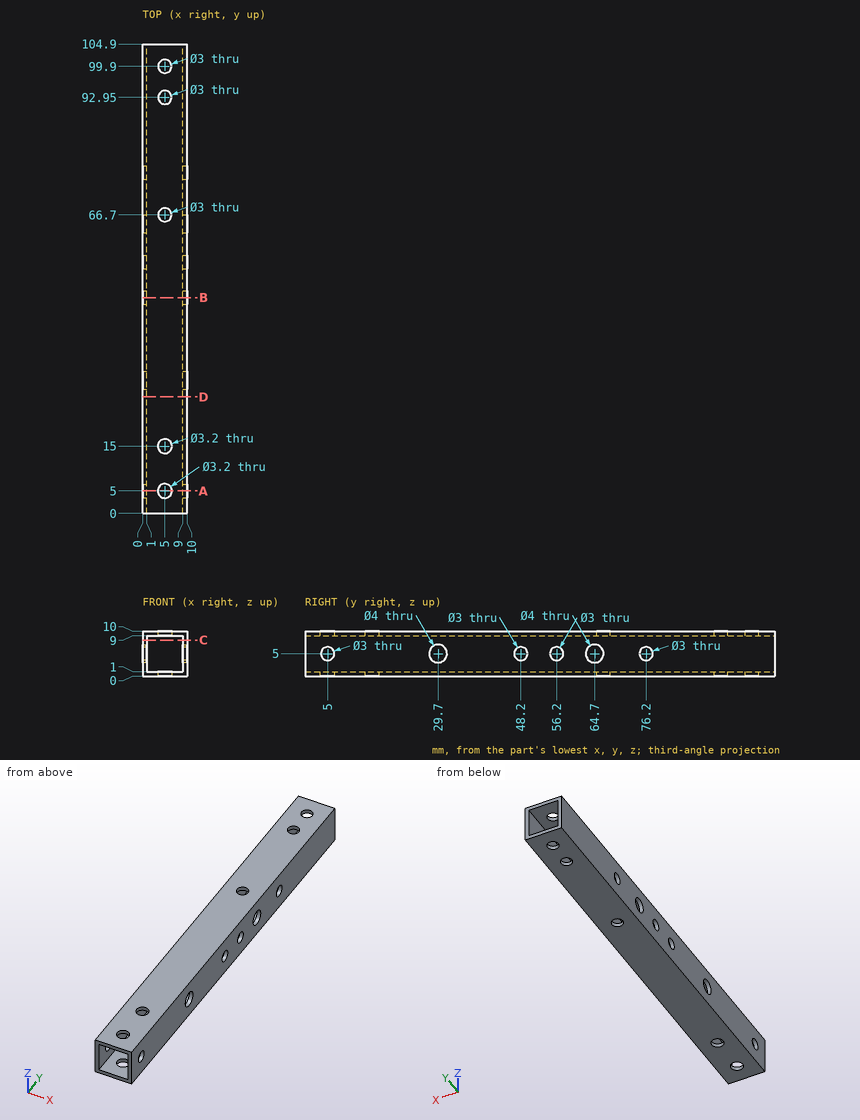
Here's the drawing with two shaded views (mm, measured from the low corner). I have some questions. Round coordinates to 2 decimals unless told otherwise and drop trailing zeros. Loops run counter-clockwise (first coordinate to the right, second up) from the corner with the lowest first, then second, coordinate; pieces in that order, holes last.
1. Will these pins go through, and if not, where does the flat tip stop? pin 1 (3.5 mm diameter, centred on x = 5, y = 92.95, fed in from -Z); pin 2 (2.5 mm diameter, centred on y = 5, z = 5, fed in from +X).
Answers:
pin 1: stops at z = 0
pin 2: passes through
2. Suppose I cut it at A-A, the plane y = 5. Please give me the cut outline in (x, z), and give its area (3 significant figures).
Answers:
outline: (0, 0) - (3.4, 0) - (3.4, 1) - (1, 1) - (1, 3.5) - (0, 3.5) - close; (0, 6.5) - (1, 6.5) - (1, 9) - (3.4, 9) - (3.4, 10) - (0, 10) - close; (6.6, 0) - (10, 0) - (10, 3.5) - (9, 3.5) - (9, 1) - (6.6, 1) - close; (6.6, 9) - (9, 9) - (9, 6.5) - (10, 6.5) - (10, 10) - (6.6, 10) - close
area: 23.6 mm2
3. Suppose I cut it at D-D, the plane y = 26. Please give me the cut outline in (x, z), and give its area (3 significant figures).
Answers:
outline: (0, 0) - (10, 0) - (10, 10) - (0, 10) - close; hole (1, 1) - (9, 1) - (9, 9) - (1, 9) - close
area: 36.0 mm2
4. Suppose I cut it at B-B, the plane y = 48.2. Please give me the cut outline in (x, z).
Answers:
outline: (0, 0) - (10, 0) - (10, 3.5) - (9, 3.5) - (9, 1) - (1, 1) - (1, 3.5) - (0, 3.5) - close; (0, 6.5) - (1, 6.5) - (1, 9) - (9, 9) - (9, 6.5) - (10, 6.5) - (10, 10) - (0, 10) - close
5. Suppose I cut it at C-C, the plane z = 8. Please give me the cut outline in (x, y).
Answers:
outline: (0, 0) - (1, 0) - (1, 104.9) - (0, 104.9) - close; (9, 0) - (10, 0) - (10, 104.9) - (9, 104.9) - close
6. If I drill on probe 1 along Z at (x, y) = (1.5, 57.5); probe 2 along X at (y, z) = (99.9, 9.25), over which ranges is the centre line in solid material (lowest first)?
Answers:
probe 1: z = 0 to 1, 9 to 10
probe 2: x = 0 to 3.5, 6.5 to 10
